Design review of the part shown in the three views and the two pictorial views. Dimensions are in mm from the part's minimum x, y and z. Give positions to 0.01 mm unless a question says otherwise; leave off trailing zeros. Loops run counter-clockwise (first coordinate to the right, second up) from the corner with the lowest first, then second, coordinate; pieces in that order, holes last. Notation, with made-up numbers: (70.25, 53) - (121.25, 53) arc R16 ccw to (121.25, 77) - close; hole circle Ø8 at (68.5, 21). An arc over 180 degrees is marked (long way). Answer in a Markdown table with one row per item.
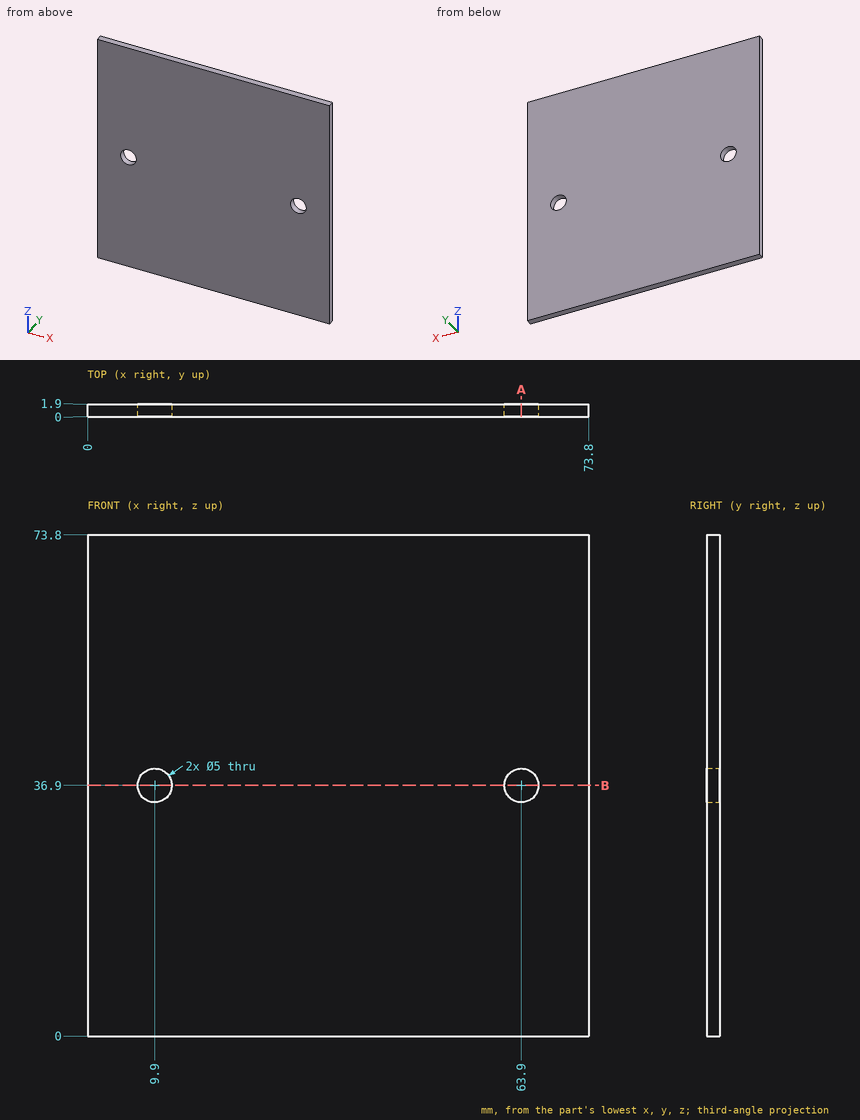
1. We need section A-A, the plane x = 63.9. Give the boundary of the cut face in (y, z).
Values:
| item | result |
|---|---|
| outline | (0, 0) - (1.9, 0) - (1.9, 34.4) - (0, 34.4) - close; (0, 39.4) - (1.9, 39.4) - (1.9, 73.8) - (0, 73.8) - close |
2. Clearance check with flat-ended pins moving along their axes: pin 1 (1 mm diameter, centred on x = 50, y = 1.5, fed in from -Z); pin 2 (4 mm diameter, centred on x = 9.9, z = 36.9, fed in from -Y). State where each tip first meets the part, or that it passes through.
Values:
| item | result |
|---|---|
| pin 1 | stops at z = 0 |
| pin 2 | passes through |
3. We need section B-B, the plane z = 36.9. Give the boundary of the cut face in (x, y), and give its area (3 significant figures).
Values:
| item | result |
|---|---|
| outline | (0, 0) - (7.4, 0) - (7.4, 1.9) - (0, 1.9) - close; (12.4, 0) - (61.4, 0) - (61.4, 1.9) - (12.4, 1.9) - close; (66.4, 0) - (73.8, 0) - (73.8, 1.9) - (66.4, 1.9) - close |
| area | 121 mm^2 |
4. Wall thickness on line 1 (X direction, y = 0.7, z = 36.9); line 2 (Z direction, x = 9.9, y = 1); line 3 (Z direction, x = 62, y = 0.1): over which ranges is each line inside the solid? List them lowest first. Write a range as [from, to].
Values:
| item | result |
|---|---|
| line 1 | x = [0, 7.4], [12.4, 61.4], [66.4, 73.8] |
| line 2 | z = [0, 34.4], [39.4, 73.8] |
| line 3 | z = [0, 35.28], [38.52, 73.8] |
